from build123d import *

# Parameters (mm, degrees)
F1_DEPTH = 5
F2_R     = 2
F3_R     = 0.4


with BuildPart() as f1:
    # F0 (on Top) → F1 (new body)
    with BuildSketch(Plane.XY):
        with BuildLine():
            Line((49.969541, 1.744975), (0, 0))
            Line((0, 0), (0, 33.9))
            Line((0, 33.9), (60, 33.9))
            Line((60, 33.9), (60, 38.9))
            Line((60, 38.9), (58.471325, 43.1))
            Line((58.471325, 43.1), (57.053565, 43.1))
            ThreePointArc((57.053565, 43.1), (56, 39.4), (54.946435, 43.1))
            Line((54.946435, 43.1), (49.053565, 43.1))
            ThreePointArc((49.053565, 43.1), (48, 39.4), (46.946435, 43.1))
            Line((46.946435, 43.1), (41.053565, 43.1))
            ThreePointArc((41.053565, 43.1), (40, 39.4), (38.946435, 43.1))
            Line((38.946435, 43.1), (33.053565, 43.1))
            ThreePointArc((33.053565, 43.1), (32, 39.4), (30.946435, 43.1))
            Line((30.946435, 43.1), (25.8, 43.1))
            ThreePointArc((25.8, 43.1), (24, 37.7), (22.2, 43.1))
            Line((22.2, 43.1), (17.8, 43.1))
            ThreePointArc((17.8, 43.1), (16, 37.7), (14.2, 43.1))
            Line((14.2, 43.1), (9.8, 43.1))
            ThreePointArc((9.8, 43.1), (8, 37.7), (6.2, 43.1))
            Line((6.2, 43.1), (1.8, 43.1))
            ThreePointArc((1.8, 43.1), (0, 37.7), (-1.8, 43.1))
            Line((-1.8, 43.1), (-3.471325, 43.1))
            Line((-3.471325, 43.1), (-5, 38.9))
            Line((-5, 38.9), (-5, -5.177652))
            Line((-5, -5.177652), (49.969541, -3.258073))
            Line((49.969541, -3.258073), (49.969541, 1.744975))
        make_face()
    extrude(amount=F1_DEPTH)

    # F2
    f2_edges = [f1.edges().sort_by_distance(p)[0] for p in [
        (49.969541, 1.744975, 2.5),
        (49.969541, -3.258073, 2.5),
        (-5, -5.177652, 2.5),
        (-5, 38.9, 2.5),
        (60, 33.9, 2.5),
        (60, 38.9, 2.5),
    ]]
    fillet(f2_edges, radius=F2_R)

    # F3
    f3_edges = [f1.edges().sort_by_distance(p)[0] for p in [
        (-1.8, 43.1, 2.5),
        (-3.471325, 43.1, 2.5),
        (-2.635663, 43.1, 0),
        (-2.635663, 43.1, 5),
        (6.2, 43.1, 2.5),
        (1.8, 43.1, 2.5),
        (4, 43.1, 0),
        (4, 43.1, 5),
        (14.2, 43.1, 2.5),
        (9.8, 43.1, 2.5),
        (12, 43.1, 0),
        (12, 43.1, 5),
        (22.2, 43.1, 2.5),
        (17.8, 43.1, 2.5),
        (20, 43.1, 0),
        (20, 43.1, 5),
        (30.946435, 43.1, 2.5),
        (25.8, 43.1, 2.5),
        (28.373217, 43.1, 0),
        (28.373217, 43.1, 5),
        (38.946435, 43.1, 2.5),
        (33.053565, 43.1, 2.5),
        (36, 43.1, 0),
        (36, 43.1, 5),
        (46.946435, 43.1, 2.5),
        (41.053565, 43.1, 2.5),
        (44, 43.1, 0),
        (44, 43.1, 5),
        (54.946435, 43.1, 2.5),
        (49.053565, 43.1, 2.5),
        (52, 43.1, 0),
        (52, 43.1, 5),
        (58.471325, 43.1, 2.5),
        (57.053565, 43.1, 2.5),
        (57.762445, 43.1, 0),
        (57.762445, 43.1, 5),
    ]]
    fillet(f3_edges, radius=F3_R)


solid = f1.part
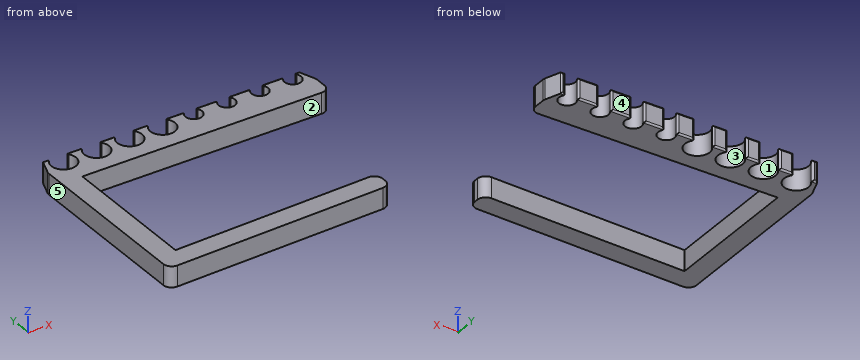
Verification items for the finished model (mm, model axes). Face numbers are marked on the shaded views. A direction names the side the tool comes from. Give positions to 0.01 mm unless a question says otherwise; leave off trailing zeros. Order: outer loops, then holes, each group sorted by start corner. A loop starts at its lowest first (then second) coordinate and runs counter-clockwise, first axis right, second up. Notation, with made-up numbers: M -8,56.5 L 32,56.5 A18 ccw 32,87.5 Z; hole C 42.25,72.25 d5. An arc over 180 degrees is marked long. Answer as a JSON object with one key per item and string values. Group by question number.
1) Cross-section at D-D (x = 8). Enter the section's corners in (y, z).
2) Mould release check, pull along Y, two halves, no side actions. Record for the marked faces 3, 4 and 5: released by +Y, released by -Y, zero draft, split by the parting line, or undercut.
3) Depth check by flat-ended pin: pin 1 Ø3 at (x, z) = (41, 0.5) entering from +Y; pin 2 Ø0.8 at (y, z) = (-1, 3) entering from +X; pin 3 Ø2.5 at (x, y) = (32, 41.4) entering from +Z; pin 4 Ø1.5 at (y, z) = (14, 1.5) entering from +X. Enter the tip coordinate at first touch or a pass-through.
4) Cross-section at A-A (x = 32). Enter the section's corners in (y, z), then the cut area to 3 significant figures.
5) Access from +Z, -Z, +X, -X, +Y, -Y to the whole of each face (thin tool, end or side, straight path). Record for the marked faces 1 and 2.
6) Cross-section at C-C (y = 7.5). Enter the section's corners in (x, z).
7) Scan lines: line 1 along X through (y, z) = (39, 0.8); line 2 along X through (y, z) = (29, 4.15); line 3 along Y through (x, z) = (44.5, 3.65). Record each from-to range of solid material in increasing order. Write a range as [from, to].
8) Cross-section at B-B (y = 41.4). Give the number of separate pieces and of enclosed holes in the cut face, then the cut area to 3 significant figures.
Result sheet:
{
 "1": {"outline": "M -4.72,0 L 0.28,0 L 0.28,5 L -4.72,5 Z; M 33.9,0 L 37.7,0 L 37.7,5 L 33.9,5 Z"},
 "2": {"face 3": "undercut", "face 4": "released by +Y", "face 5": "zero draft"},
 "3": {"pin 1": "stops at y = 43.1", "pin 2": "stops at x = 49.97", "pin 3": "passes through", "pin 4": "stops at x = 0"},
 "4": {"outline": "M -3.89,0 L 1.12,0 L 1.12,5 L -3.89,5 Z; M 33.9,0 L 39.4,0 L 39.4,5 L 33.9,5 Z", "area": "52.5 mm2"},
 "5": {"face 1": "+Z, -Z", "face 2": "+Z, -Z, +X"},
 "6": {"outline": "M -5,0 L 0,0 L 0,5 L -5,5 Z"},
 "7": {"line 1": "x = [-4.95, -2.47], [2.47, 5.53], [10.47, 13.53], [18.47, 21.53], [26.47, 59.95]", "line 2": "x = [-5, 0]", "line 3": "y = [-3.45, 1.55], [33.9, 43.1]"},
 "8": {"separate pieces": "9", "enclosed holes": "0", "area": "119 mm2"}
}
